The drawing under review shows one solid part. Ordinate dimensions are in mm from its lowest x, y, z. Round coordinates to 2 decimals unless told otherwise and drop trailing zeros. Write each loop counter-clockwise with the first axis right and the second up, starting at its lowest first coordinate (ties: lowest second). Pieces come first, ordered by that corner, then holes. Notation, with made-up numbers: (17, 54.25) -> (66, 54.25) arc R21 ccw to (66, 85.25) -> close; hole circle Ø3 at (-17, 80). An arc over 180 degrees is marked (long way). Write item = value, one per line. Start each with the question number.
Item 1: Add section C-C, the plane z = 0.85. State the section outline as (x, y) points (1 decimal).
Item 2: Add section B-B, the plane x = 42.5. State the section outline as (y, z) points.
Item 3: For pin 1 Ø11 at (x, y) = (76.375, 42.5) entering from -Z, flat-tipped, find the tip position at first contact; note if it passes through.
Item 4: To check wall thickness, follow L1, parallel to Y at x = 60.5, z = 0.75; L2, parallel to Y at x = 43, z = 0.85 (1 decimal); L3, parallel to X at y = 70.5, z = 0.45 (1 decimal). State the ranges of each line that lie inside material, in increasing order.
Item 5: Add section A-A, the plane y = 42.5. State the section outline as (x, z) points (1 decimal), then the cut area to 3 significant figures.
Item 6: Add section D-D, the plane y = 19. State the section outline as (x, z) points.
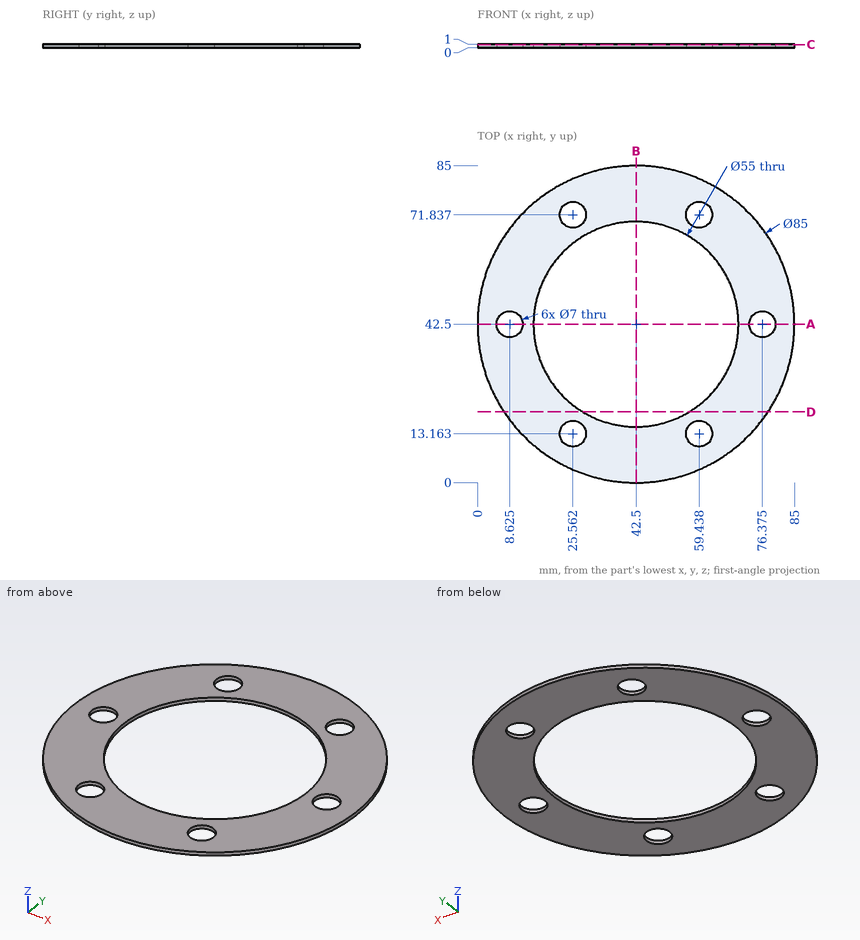
Result set:
q1.outline = circle Ø85 at (42.5, 42.5); hole circle Ø7 at (8.6, 42.5); hole circle Ø55 at (42.5, 42.5); hole circle Ø7 at (25.6, 13.2); hole circle Ø7 at (25.6, 71.8); hole circle Ø7 at (59.4, 13.2); hole circle Ø7 at (59.4, 71.8); hole circle Ø7 at (76.4, 42.5)
q2.outline = (0, 0) -> (15, 0) -> (15, 1) -> (0, 1) -> close; (70, 0) -> (85, 0) -> (85, 1) -> (70, 1) -> close
q3.pin_1 = 0
q4.L1 = 4 to 9.83, 16.5 to 21.71, 63.29 to 68.5, 75.17 to 81
q4.L2 = 0 to 15, 70 to 85
q4.L3 = 10.5 to 22.3, 28.8 to 56.2, 62.7 to 74.5
q5.outline = (0, 0) -> (5.1, 0) -> (5.1, 1) -> (0, 1) -> close; (12.1, 0) -> (15, 0) -> (15, 1) -> (12.1, 1) -> close; (70, 0) -> (72.9, 0) -> (72.9, 1) -> (70, 1) -> close; (79.9, 0) -> (85, 0) -> (85, 1) -> (79.9, 1) -> close
q5.area = 16.0 mm²
q6.outline = (7.09, 0) -> (28.22, 0) -> (28.22, 1) -> (7.09, 1) -> close; (56.78, 0) -> (77.91, 0) -> (77.91, 1) -> (56.78, 1) -> close
